Here's how the part is built. I have some questions about the finished solid (model axes, mm). A direction names the side the tool comes from. Coordinates: 2 decimals unless noted, no trailing zeros. Loops run counter-clockwise (first coordinate to the right, second up) from the corner with the lowest first, then second, coordinate; pieces in that order, holes last. Notation, with made-up numbers: M -3,77.25 L 25,77.25 A17 cw 25,89.25 Z; hole C -19.75,0 d8. An arc over 180 degrees is marked long. Use one line per item in the form item = value. Start each with the question number.
(1) Imagine slicing it at A-A, the plane x = 86.5. Please give me the cut outline in (y, z).
(2) Imagine slicing it at B-B, the plane z = 2.15. Please give me the cut outline in (x, y).
(3) Please list where these lines run through material, in increasing order: L1, parallel to Y at x = 11, z = 4.75; L2, parallel to X at y = 83, z = 1.6; L3, parallel to X at y = 11.5, z = 0.55.
(4) On a 3-axis mill with a long thin cutter (end or side, diameter ignored), from which of +Z, -Z, +X, -X, +Y, -Y can I reach the whole of each face in a straight line? I mean faces 4 (the flat face through (38.077, 4.93, 2.535)), 5 (the flat face through (15, 48.967, 3)), 6 (the flat face through (49.378, 85, 3)). Say none if no direction works.
(5) Thinking about a two-plate mould opening in Y: for faces 1 (the cylindrical face through (52.4, 77, 2.5)), 2 (the flat face through (0, 23, 2)), 3 (the cylindrical face through (77, 42.5, 2.5)), which applies, +Y half, -Y half, draft (parallel to the pull), parting line (faces both ways), or undercut?
```python
from build123d import *

# Parameters (mm, degrees)
SKIZZE1_W                        = 100
SKIZZE1_H                        = 100
AUFSATZ_LINEAR_AUSTRAGEN1_DEPTH  = 5
SCHNITT_LINEAR_AUSTRAGEN1_REACH  = 7
SCHNITT_LINEAR_AUSTRAGEN14_REACH = 7
SCHNITT_LINEAR_AUSTRAGEN15_REACH = 7
SCHNITT_LINEAR_AUSTRAGEN16_REACH = 7


with BuildPart() as part:
    # Skizze1 → Aufsatz-Linear austragen1 (new body)
    with BuildSketch(Plane.XY):
        with Locations((50, 50)):
            Rectangle(SKIZZE1_W, SKIZZE1_H)
    extrude(amount=AUFSATZ_LINEAR_AUSTRAGEN1_DEPTH)

    # Skizze2 → Schnitt-Linear austragen1 (cut, up to next)
    with BuildSketch(Plane(origin=(61.541641428, 22.675716927, 5), x_dir=(1, 0, 0), z_dir=(0, 0, 1)), mode=Mode.PRIVATE) as schnitt_linear_austragen1_sk1:
        with BuildLine():
            Line((-24.45087326, -22.675716927), (-22.45087326, -12.675716927))
            Line((-22.45087326, -12.675716927), (-22.45087326, -2.675716927))
            ThreePointArc((-22.45087326, -2.675716927), (-19.45087326, 0.324283073), (-16.45087326, -2.675716927))
            Line((-16.45087326, -2.675716927), (-16.45087326, -12.675716927))
            Line((-16.45087326, -12.675716927), (-14.45087326, -22.675716927))
            Line((-14.45087326, -22.675716927), (-24.45087326, -22.675716927))
        make_face()
    schnitt_linear_austragen1_tool1 = extrude(schnitt_linear_austragen1_sk1.sketch, amount=-SCHNITT_LINEAR_AUSTRAGEN1_REACH, mode=Mode.PRIVATE) & part.part
    add(schnitt_linear_austragen1_tool1.solids().sort_by_distance((42.090768, 10.16893, 5))[0], mode=Mode.SUBTRACT)

    # Skizze24 → Schnitt-Linear austragen14 (cut, up to next)
    with BuildSketch(Plane(origin=(44.055881927, 74.466743066, 5), x_dir=(1, 0, 0), z_dir=(0, 0, 1)), mode=Mode.PRIVATE) as schnitt_linear_austragen14_sk1:
        with BuildLine():
            Line((-44.055881927, -17.5), (-34.055881927, -19.5))
            Line((-34.055881927, -19.5), (-24.055881927, -19.5))
            ThreePointArc((-24.055881927, -19.5), (-21.055881927, -22.5), (-24.055881927, -25.5))
            Line((-24.055881927, -25.5), (-34.055881927, -25.5))
            Line((-34.055881927, -25.5), (-44.055881927, -27.5))
            Line((-44.055881927, -27.5), (-44.055881927, -17.5))
        make_face()
    schnitt_linear_austragen14_tool1 = extrude(schnitt_linear_austragen14_sk1.sketch, amount=-SCHNITT_LINEAR_AUSTRAGEN14_REACH, mode=Mode.PRIVATE) & part.part
    add(schnitt_linear_austragen14_tool1.solids().sort_by_distance((10.16893, 51.966743, 5))[0], mode=Mode.SUBTRACT)

    # Skizze25 → Schnitt-Linear austragen15 (cut, up to next)
    with BuildSketch(Plane(origin=(81.625168415, 83.365494521, 5), x_dir=(1, 0, 0), z_dir=(0, 0, 1)), mode=Mode.PRIVATE) as schnitt_linear_austragen15_sk1:
        with BuildLine():
            Line((-24.247626507, 16.634505479), (-26.247626507, 6.634505479))
            Line((-26.247626507, 6.634505479), (-26.247626507, -3.365494521))
            ThreePointArc((-26.247626507, -3.365494521), (-29.247626507, -6.365494521), (-32.247626507, -3.365494521))
            Line((-32.247626507, -3.365494521), (-32.247626507, 6.634505479))
            Line((-32.247626507, 6.634505479), (-34.247626507, 16.634505479))
            Line((-34.247626507, 16.634505479), (-24.247626507, 16.634505479))
        make_face()
    schnitt_linear_austragen15_tool1 = extrude(schnitt_linear_austragen15_sk1.sketch, amount=-SCHNITT_LINEAR_AUSTRAGEN15_REACH, mode=Mode.PRIVATE) & part.part
    add(schnitt_linear_austragen15_tool1.solids().sort_by_distance((52.377542, 89.83107, 5))[0], mode=Mode.SUBTRACT)

    # Skizze26 → Schnitt-Linear austragen16 (cut, up to next)
    with BuildSketch(Plane(origin=(95.870397917, 55.045051389, 5), x_dir=(1, 0, 0), z_dir=(0, 0, 1)), mode=Mode.PRIVATE) as schnitt_linear_austragen16_sk1:
        with BuildLine():
            Line((4.129602083, -17.5), (-5.870397917, -15.5))
            Line((-5.870397917, -15.5), (-15.870397917, -15.5))
            ThreePointArc((-15.870397917, -15.5), (-18.870397917, -12.5), (-15.870397917, -9.5))
            Line((-15.870397917, -9.5), (-5.870397917, -9.5))
            Line((-5.870397917, -9.5), (4.129602083, -7.5))
            Line((4.129602083, -7.5), (4.129602083, -17.5))
        make_face()
    schnitt_linear_austragen16_tool1 = extrude(schnitt_linear_austragen16_sk1.sketch, amount=-SCHNITT_LINEAR_AUSTRAGEN16_REACH, mode=Mode.PRIVATE) & part.part
    add(schnitt_linear_austragen16_tool1.solids().sort_by_distance((89.83107, 42.545051, 5))[0], mode=Mode.SUBTRACT)


solid = part.part
```
Answer:
q1.outline = M 0,0 L 39.55,0 L 39.55,5 L 0,5 Z; M 45.55,0 L 100,0 L 100,5 L 45.55,5 Z
q2.outline = M 0,0 L 37.09,0 L 39.09,10 L 39.09,20 A3 cw 45.09,20 L 45.09,10 L 47.09,0 L 100,0 L 100,37.55 L 90,39.55 L 80,39.55 A3 cw 80,45.55 L 90,45.55 L 100,47.55 L 100,100 L 57.38,100 L 55.38,90 L 55.38,80 A3 cw 49.38,80 L 49.38,90 L 47.38,100 L 0,100 L 0,56.97 L 10,54.97 L 20,54.97 A3 cw 20,48.97 L 10,48.97 L 0,46.97 Z
q3.L1 = 0 to 48.97, 54.97 to 100
q3.L2 = 0 to 49.38, 55.38 to 100
q3.L3 = 0 to 39.09, 45.09 to 100
q4.face_4 = +Z, -Z, -Y
q4.face_5 = +Z, -Z, -X
q4.face_6 = +Z, -Z, +Y
q5.face_1 = +Y half
q5.face_2 = draft
q5.face_3 = undercut
